The listing builds one solid part. Answer for the finished solid, in the listing's coordinates (mm). A direction names the side the tool comes from. Coordinates: 2 decimals unless noted, no trailing zeros. Loops run counter-clockwise (first coordinate to the right, second up) from the corner with the lowest first, then second, coordinate; pieces in that order, holes last. Notation, with made-up numbers: M 34,33 L 75,33 A19 ccw 75,57 Z; hole C -21,-17 d7. An arc over 180 degrees is marked long. Answer as a JSON object with one key per item and string values. Group by question number.
1. Given pin 1 (10.5 mm diameter, centred on x = 33, z = 15, fed in from +Y); pin 2 (11 mm diameter, centred on x = 26, y = -6.5, fed in from -Z); pin 3 (15 mm diameter, centred on x = 14, z = 12.5, fed in from -Y); pin 4 (4 mm diameter, centred on x = 33, z = 15, fed in from +Y), each flat-ended and moving along its own axis, determine where each tip first touches the part or whether it passes through.
2. For faces 4 (the face through (22.5, 18, 15)), 5 (the face through (26, -4, 10)), 6 (the face through (26, -4, 20)), 7 (the face through (26.19, -3.61, 15.07)), 8 (the face through (15, 3, 15)), determine the directions among +Z, -Z, +X, -X, +Y, -Y from which every point of the face is accessible in a straight line to the end or side of a thin tool.
3. A cutting plane is placed at D-D on z = 15. State how many separate pieces and enclosed holes the cut face has, and give its area (3 significant figures).
4. Determine the mould class of faces 1 (the face through (0, 2, 15)), 2 (the face through (9.5, 15, 15)), 3 (the face through (20, 9, 0)) for opening direction X: released by +X, released by -X, zero draft, split by the parting line, or undercut.
5. A cutting plane is placed at A-A on y = 10. Give the vertices of the cut face in (x, z), and give its area (3 significant figures).
6. A cutting plane is placed at B-B on x = 33. Give the vertices of the cut face in (y, z).
7. A cutting plane is placed at C-C on z = 26. Give the vertices of the cut face in (x, y), and give its area (3 significant figures).
8. Straight lines are drawn through the part: L1, parallel to Z at x = 33, y = -2.5; L2, parallel to X at y = 25, z = 25; L3, parallel to X at y = 0.85, z = 15. For each, find the intervals that lie inside material, in ascending order.
from build123d import *

# Parameters (mm, degrees)
BOSS_EXTRU_1_DEPTH      = 30
ESQUISSE2_R             = 3.25
ENL_V_MAT_EXTRU_1_DEPTH = 56.901699437
ESQUISSE3_R             = 5.25
ESQUISSE3_R_2           = 3.25
EXTRU_MINCE1_DEPTH      = 10
ESQUISSE5_W             = 3
ESQUISSE5_H             = 25
BOSS_EXTRU_3_DEPTH      = 30
CONG_1_R                = 5
CONG_2_R                = 2
EXTRU_MINCE2_START      = -10
EXTRU_MINCE2_DEPTH      = 10


with BuildPart() as part:
    # Esquisse1 → Boss.-Extru.1 (new body)
    with BuildSketch(Plane.XY):
        with BuildLine():
            Line((0, 0), (40, 0))
            Line((40, 0), (40, 3))
            Line((40, 3), (9.5, 3))
            Line((9.5, 3), (9.5, 28))
            Line((9.5, 28), (5.5, 28))
            Line((5.5, 28), (5.5, 8))
            ThreePointArc((5.5, 8), (4.035533906, 4.464466094), (0.5, 3))
            Line((0.5, 3), (0, 3))
            Line((0, 3), (0, 0))
        make_face()
    extrude(amount=BOSS_EXTRU_1_DEPTH)

    # Esquisse2 → Enlèv. mat.-Extru.1 (cut, through all)
    with BuildSketch(Plane(origin=(0, 3, 0), x_dir=(1, 0, 0), z_dir=(0, 1, 0))):
        with Locations(Location((33, -15, 0), (0, 0, 270))):
            Circle(ESQUISSE2_R)
    extrude(amount=-ENL_V_MAT_EXTRU_1_DEPTH, mode=Mode.SUBTRACT)

    # Esquisse3 → Extru.-Mince1 (add)
    with BuildSketch(Plane(origin=(0, 0, 0), x_dir=(-1, 0, 0), z_dir=(0, -1, 0))):
        with Locations((-33, -15)):
            Circle(ESQUISSE3_R)
        with Locations((-33, -15)):
            Circle(ESQUISSE3_R_2, mode=Mode.SUBTRACT)
    extrude(amount=EXTRU_MINCE1_DEPTH)

    # Esquisse5 → Boss.-Extru.3 (add)
    with BuildSketch(Plane.XY.offset(30)):
        with Locations((21, 15.5)):
            Rectangle(ESQUISSE5_W, ESQUISSE5_H)
    extrude(amount=-BOSS_EXTRU_3_DEPTH)

    # Congé1
    cong_1_edges = [part.edges().sort_by_distance(p)[0] for p in [
        (22.5, 3, 15),
    ]]
    fillet(cong_1_edges, radius=CONG_1_R)

    # Congé2
    cong_2_edges = [part.edges().sort_by_distance(p)[0] for p in [
        (38.25, 0, 15),
    ]]
    fillet(cong_2_edges, radius=CONG_2_R)

    # Esquisse6 → Extru.-Mince2 (add)
    with BuildSketch(Plane.XY.offset(30).offset(EXTRU_MINCE2_START)):
        Polygon((29.75, -10), (19.75, 0), (29.75, 0), align=None)
        Polygon((27.75, -5.171572875), (24.578427125, -2), (27.75, -2), align=None, mode=Mode.SUBTRACT)
    extrude(amount=-EXTRU_MINCE2_DEPTH)


solid = part.part
From the geometry:
{
 "1": {"pin 1": "stops at y = 3", "pin 2": "stops at z = 9.97", "pin 3": "stops at y = -1.75", "pin 4": "passes through"},
 "2": {"face 4": "+Z, -Z, +X, +Y", "face 5": "-Z, -X, -Y", "face 6": "+Z, -X, -Y", "face 7": "+Z, -Z", "face 8": "+Z, -Z, +Y"},
 "3": {"separate pieces": "2", "enclosed holes": "1", "area": "354 mm²"},
 "4": {"face 1": "released by -X", "face 2": "undercut", "face 3": "zero draft"},
 "5": {"outline": "M 5.5,0 L 9.5,0 L 9.5,30 L 5.5,30 Z; M 19.5,0 L 22.5,0 L 22.5,30 L 19.5,30 Z", "area": "210 mm²"},
 "6": {"outline": "M -10,9.75 L -2,9.75 A2 cw 0,7.75 L 0,0 L 3,0 L 3,11.75 L -10,11.75 Z; M -10,18.25 L 3,18.25 L 3,30 L 0,30 L 0,22.25 A2 cw -2,20.25 L -10,20.25 Z"},
 "7": {"outline": "M 0,0 L 40,0 L 40,3 L 27.5,3 A5 cw 22.5,8 L 22.5,28 L 19.5,28 L 19.5,3 L 9.5,3 L 9.5,28 L 5.5,28 L 5.5,8 A5 cw 0.5,3 L 0,3 Z", "area": "306 mm²"},
 "8": {"L1": "z = 9.75 to 11.75, 18.25 to 20.25", "L2": "x = 5.5 to 9.5, 19.5 to 22.5", "L3": "x = 0 to 29.75, 36.25 to 40"}
}
